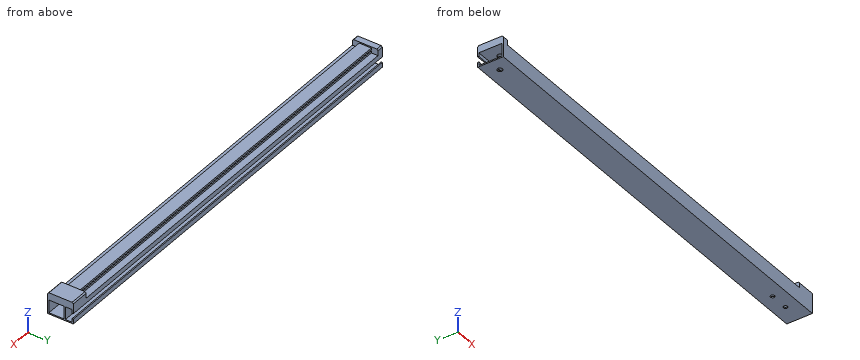
Autodesk Inventor part; units mm, degrees
ref_plane "YZ Plane" through (0, 0, 0) normal (1, 0, 0) x (0, 1, 0)
ref_plane "XZ Plane" through (0, 0, 0) normal (0, 1, 0) x (-1, 0, 0)
ref_plane "XY Plane" through (0, 0, 0) normal (0, 0, 1) x (1, 0, 0)
sketch "草图1" plane through (0, 0, 0) normal (1, 0, 0) x (0, 1, 0)
  line L0 (21, 12.5) -> (-21, 12.5)
  line L1 (-21, 12.5) -> (-21, -12.5)
  line L2 (-21, -12.5) -> (21, -12.5)
  line L3 (21, 12.5) -> (-21, -12.5) construction
  line L4 (-21, 12.5) -> (21, -12.5) construction
  line L5 (19, 10.5) -> (-19, 10.5)
  line L6 (-19, 10.5) -> (-19, -10.5)
  line L7 (-19, -10.5) -> (19, -10.5)
  line L8 (21, 4.5) -> (19, 4.5)
  line L9 (21, -4.5) -> (19, -4.5)
  line L10 (21, -12.5) -> (21, -4.5)
  line L11 (21, 4.5) -> (21, 12.5)
  line L12 (19, -10.5) -> (19, -4.5)
  line L13 (19, 4.5) -> (19, 10.5)
  line L14 (0, 10.5) -> (-2, 10.5)
  line L15 (-2, -10.5) -> (0, -10.5)
  line L16 (8, -12.5) -> (6, -12.5)
  line L17 (6, -12.5) -> (6, 12.5)
  line L18 (6, 12.5) -> (8, 12.5)
  line L19 (8, 12.5) -> (8, -12.5)
  point P0 (0, 0)
  point P1 (6, -10.5)
  point P2 (6, 10.5)
  point P3 (8, -10.5)
  point P4 (8, 10.5)
  dimension "d0" = 42
  dimension "d1" = 25
  dimension "d3" = 8
  dimension "d4" = 8
  dimension "d9" = 2
  dimension "d10" = 25
extrude "拉伸2" add sketch "草图1" along normal blind 680 contours L11 L8 L13 L5 L19 L0 | L19 L5 L17 L0 | L17 L5 L6 L7 L2 L1 L0 | L19 L7 L17 L5 | L19 L2 L17 L7 | L7 L12 L9 L10 L2 L19
sketch "草图2" plane through (0, -19, -10.5) normal (0, 0, 1) x (1, 0, 0)
  circle A0 centre (617.3314, 19) radius 3.3235
  circle A1 centre (647.3314, 19) radius 3.3235
  point P0 (0, 19)
extrude "拉伸3" cut sketch "草图2" against normal blind 2
sketch "草图3" plane through (0, 0, 0) normal (-1, 0, 0) x (0, 0, 1)
  line L0 (-12.5, 21) -> (-4.5, 21)
  line L1 (-12.5, -21) -> (-12.5, 21)
  line L2 (12.5, -21) -> (-12.5, -21)
  line L3 (12.5, 21) -> (12.5, -21)
  line L4 (4.5, 21) -> (12.5, 21)
  line L5 (4.5, 19) -> (4.5, 21)
  line L6 (10.5, 19) -> (4.5, 19)
  line L7 (10.5, 8) -> (10.5, 19)
  line L8 (-10.5, 8) -> (10.5, 8)
  line L9 (-10.5, 19) -> (-10.5, 8)
  line L10 (-4.5, 19) -> (-10.5, 19)
  line L11 (-4.5, 21) -> (-4.5, 19)
  line L12 (-10.5, 6) -> (-10.5, -19)
  line L13 (10.5, 6) -> (-10.5, 6)
  line L14 (10.5, -19) -> (10.5, 6)
  line L15 (-10.5, -19) -> (10.5, -19)
  line L16 (-10.5, 8) -> (-10.5, 6)
  line L17 (-10.5, 8) -> (10.5, 8)
  line L18 (10.5, -19) -> (10.5, 6)
  line L19 (10.5, 8) -> (10.5, 6)
  point P0 (0, 0)
extrude "拉伸4" add sketch "草图3" along normal blind 40 contours L0 L11 L10 L9 L16 L12 L15 L14 L19 L7 L6 L5 L4 L3 L2 L1
sketch "草图4" plane through (680, -21, 12.5) normal (0, 0, 1) x (1, 0, 0)
  circle A0 centre (-698, 21) radius 4.25
  line L0 (-720, 0) -> (-720, 42)
  point P0 (-680, 21)
  dimension "d17" = 8.5
  dimension "d18" = 22
extrude "拉伸5" cut sketch "草图4" against normal blind 40
sketch "草图5" plane through (-40, 0, 0) normal (-1, 0, 0) x (0, 0, 1)
  line L0 (4.5, 21) -> (12.5, 21)
  line L1 (12.5, 21) -> (22.5, 21)
  line L2 (22.5, 21) -> (22.5, -21)
  line L3 (22.5, -21) -> (12.5, -21)
  line L4 (12.5, -21) -> (12.5, 21)
  point P0 (0, 0)
  dimension "d21" = 10
  dimension "d22" = 42
extrude "拉伸6" add sketch "草图5" against normal blind 10
chamfer "倒角1" distance 2 angle 45 2 edges at (-35, 21, 22.5) (-35, -21, 22.5)
sketch "草图6" plane through (-30, 0, 0) normal (1, 0, 0) x (0, 0, -1)
  line L0 (-12.5, 21) -> (-12.5, -21)
  line L1 (-20.5, -10) -> (-20.5, 10)
  line L2 (-12.5, 10) -> (-12.5, -10)
  line L3 (-12.5, 21) -> (-20.5, 21)
  line L4 (-15.5, -10) -> (-15.5435, -10)
  line L5 (-15.5, -10) -> (-17.5, -10)
  line L6 (-17.5, -10) -> (-17.5, -7)
  line L7 (-17.5, -7) -> (-15.5, -7)
  line L8 (-15.5, -7) -> (-15.5, -10)
  line L9 (-15.5, 10) -> (-15.5, 7)
  line L10 (-15.5, 7) -> (-17.5, 7)
  line L11 (-17.5, 7) -> (-17.5, 10)
  line L12 (-20.5, 10) -> (-17.5, 10)
  line L13 (-15.5, 10) -> (-12.5, 10)
  line L14 (-12.5, -10) -> (-15.5, -10)
  line L15 (-17.5, -10) -> (-20.5, -10)
  point P0 (0, 0)
  dimension "d30" = 8
  dimension "d31" = 3
  dimension "d32" = 2
  dimension "d35" = 2
extrude "拉伸7" add sketch "草图6" along normal blind 680 contours L0 L14 L8 L7 L6 L15 L1 L12 L11 L10 L9 L13
sketch "草图7" plane through (650, 0, 0) normal (1, 0, 0) x (0, 0, -1)
  line L0 (-15.5, 10) -> (-12.5, 10)
  line L1 (-12.5, 21) -> (-12.5, 10)
  line L2 (-12.5, 21) -> (-20.5, 21)
  line L3 (-22.5, 19) -> (-20.5, 21)
  line L4 (-22.5, 19) -> (-22.5, -19)
  line L5 (-20.5, -21) -> (-22.5, -19)
  line L6 (-20.5, -21) -> (-12.5, -21)
  line L7 (-12.5, -10) -> (-12.5, -21)
  line L8 (-12.5, -10) -> (-15.5, -10)
  line L9 (-15.5, -10) -> (-15.5, -7)
  line L10 (-15.5, -7) -> (-17.5, -7)
  line L11 (-17.5, -7) -> (-17.5, -10)
  line L12 (-17.5, -10) -> (-20.5, -10)
  line L13 (-20.5, -10) -> (-20.5, 10)
  line L14 (-20.5, 10) -> (-17.5, 10)
  line L15 (-17.5, 10) -> (-17.5, 7)
  line L16 (-17.5, 7) -> (-15.5, 7)
  line L17 (-15.5, 7) -> (-15.5, 10)
  line L18 (-12.5, 10) -> (-12.5, -10)
  line L19 (-12.5, 10) -> (-15.5, 10)
  line L20 (-15.5, 10) -> (-15.5, 7)
  line L21 (-15.5, 7) -> (-17.5, 7)
  line L22 (-17.5, 7) -> (-17.5, 10)
  line L23 (-17.5, 10) -> (-20.5, 10)
  line L24 (-20.5, 10) -> (-20.5, -10)
  line L25 (-20.5, -10) -> (-17.5, -10)
  line L26 (-17.5, -10) -> (-17.5, -7)
  line L27 (-17.5, -7) -> (-15.5, -7)
  line L28 (-15.5, -7) -> (-15.5, -10)
  line L29 (-15.5, -10) -> (-12.5, -10)
  point P0 (0, 0)
extrude "拉伸8" add sketch "草图7" along normal blind 30
properties part number "连接桥"
Input: part model. Units: mm. Frame: model coordinates. Give positions to 0.01 mm unless a question says otherwise; leave off trailing zeros. Write each loop counter-clockwise with the first axis right and the second up, starting at its lowest first coordinate (ties: lowest second). Pieces come first, ordered by that corner, then holes. Notation, with made-up numbers: (-26.75, -16) - (-19.75, -16) arc R16 ccw to (-19.75, 1) - close; hole circle Ø2 at (6.25, 4). An arc over 180 degrees is marked (long way). Write item = value, one per line. Start each with the question number.
1. Ray query, L1, parallel to Y at x = 257.5, z = 5; L2, parallel to Z at x = 524, y = -1; L3, parallel to Y at x = 121, z = -2.5. Return the intervals inside material, ascending.
2. Section query A-A, the plane x = 73. Output: boundary loops of the cut face in (y, z).
3. First-contact query: pin 1 Ø12 at (x, y) = (174.5, -18) entering from +Z; pin 2 Ø2 at (x, y) = (468.5, 3) entering from +Z; pin 3 Ø2 at (x, z) = (351, 19) entering from +Y. Flat tips, straight axial feed; report the tip coordinate or a pass-through.
Check sheet entries:
q1.L1 = -21 to -19, 6 to 8, 19 to 21
q1.L2 = -12.5 to -10.5, 10.5 to 20.5
q1.L3 = -21 to -19, 6 to 8
q2.outline = (-21, -12.5) - (21, -12.5) - (21, -4.5) - (19, -4.5) - (19, -10.5) - (8, -10.5) - (8, 10.5) - (19, 10.5) - (19, 4.5) - (21, 4.5) - (21, 12.5) - (10, 12.5) - (10, 15.5) - (7, 15.5) - (7, 17.5) - (10, 17.5) - (10, 20.5) - (-10, 20.5) - (-10, 17.5) - (-7, 17.5) - (-7, 15.5) - (-10, 15.5) - (-10, 12.5) - (-21, 12.5) - close; hole (-19, -10.5) - (6, -10.5) - (6, 10.5) - (-19, 10.5) - close
q3.pin_1 = 12.5
q3.pin_2 = 20.5
q3.pin_3 = 10
